Work out the finished part from the listing and answer in its coordinate system (mm). A direction names the side the tool comes from. Round coordinates to 2 decimals unless told otherwise and drop trailing zeros. Write each loop counter-clockwise with the first axis right and the second up, starting at its lowest first coordinate (ties: lowest second). Pieces come first, ordered by that corner, then holes.
from build123d import *

# Parameters (mm, degrees)
BOSS_EXTRUDE1_DEPTH        = 13
CUT_EXTRUDE1_DEPTH         = 71.771362109
CUT_EXTRUDE2_DEPTH         = 62.040693778
F_8_4_8_4_DIAMETER_HOLE1_D = 8.4
CHAMFER2_SIZE              = 9
CHAMFER2_SIZE2             = 8.410167494
CHAMFER3_SIZE              = 8
CHAMFER3_SIZE2             = 8.56106612
SKETCH11_R                 = 4.2
CUT_EXTRUDE5_DEPTH         = 10
CHAMFER4_SIZE              = 0.5
SKETCH12_W                 = 893.834484117
SKETCH12_H                 = 134.722779032
CUT_EXTRUDE6_DEPTH         = 73.047156948


with BuildPart() as part:
    # Sketch1 → Boss-Extrude1 (new body)
    with BuildSketch(Plane(origin=(0, 0, 0), x_dir=(-1, 0, 0), z_dir=(0, 0, -1))):
        with BuildLine():
            Line((-14.999999535, -11.339745693), (-14.999999535, -27.999999731))
            ThreePointArc((-14.999999535, -27.999999731), (4.65e-07, -42.999999731), (15.000000465, -27.999999731))
            Line((15.000000465, -27.999999731), (15.000000465, -13.660253769))
            ThreePointArc((15.000000465, -13.660253769), (16.160254503, -9.33012675), (19.330127484, -6.160253769))
            Line((19.330127484, -6.160253769), (31.748711306, 1.009618943))
            ThreePointArc((31.748711306, 1.009618943), (37.239092363, 6.5), (39.248711306, 14))
            ThreePointArc((39.248711306, 14), (39.245992383, 14.285587643), (39.237836599, 14.571071754))
            Line((39.237836599, 14.571071754), (56.327549631, 24.437822174))
            Line((56.327549631, 24.437822174), (52.827549631, 30.5))
            Line((52.827549631, 30.5), (49.327549631, 36.562177826))
            Line((49.327549631, 36.562177826), (32.237836599, 26.695427407))
            ThreePointArc((32.237836599, 26.695427407), (31.994677998, 26.845232579), (31.748711306, 26.990381057))
            ThreePointArc((31.748711306, 26.990381057), (24.248711306, 29), (16.748711306, 26.990381057))
            Line((16.748711306, 26.990381057), (2.320508541, 18.660254307))
            ThreePointArc((2.320508541, 18.660254307), (-10.358983383, 5.980762382), (-14.999999535, -11.339745693))
        make_face()
    extrude(amount=-BOSS_EXTRUDE1_DEPTH)

    # Sketch2 → Cut-Extrude1 (cut, through all)
    with BuildSketch(Plane(origin=(-7.5, -12.990381057, 0), x_dir=(0.8660254037844388, -0.4999999999999997, 0), z_dir=(-0.4999999999999997, -0.8660254037844388, 0))):
        with BuildLine():
            ThreePointArc((-25.021227161, 9.417565156), (-22, 2.3), (-18.978772839, 9.417565156))
            ThreePointArc((-18.978772839, 9.417565156), (-22, 10.7), (-25.021227161, 9.417565156))
        make_face()
    extrude(amount=-CUT_EXTRUDE1_DEPTH, mode=Mode.SUBTRACT)

    # Sketch3 → Cut-Extrude2 (cut, through all)
    with BuildSketch(Plane.ZY.offset(15.000000465)):
        with BuildLine():
            ThreePointArc((9.417565156, -18.978772839), (2.3, -22), (9.417565156, -25.021227161))
            ThreePointArc((9.417565156, -25.021227161), (10.7, -22), (9.417565156, -18.978772839))
        make_face()
    extrude(amount=-CUT_EXTRUDE2_DEPTH, mode=Mode.SUBTRACT)

    # Ø8.4 (8.4) Diameter Hole1 (through all)
    with Locations(Plane(origin=(0, 0, 0), x_dir=(-1, 0, 0), z_dir=(0, 0, -1))):
        with Locations((29.347432097, 16.831243464), (0.097432097, -33.831242658)):
            Hole(F_8_4_8_4_DIAMETER_HOLE1_D / 2)

    # Chamfer2
    chamfer2_edges = [part.edges().sort_by_distance(p)[0] for p in [
        (-40.782693115, 31.628802617, 0),
    ]]
    chamfer2_side = [part.faces().sort_by_distance(p)[0] for p in [
        (-40.782693115, 31.628802617, 6.5),
    ]]
    chamfer(chamfer2_edges, length=CHAMFER2_SIZE, length2=CHAMFER2_SIZE2, reference=chamfer2_side[0])

    # Chamfer3
    chamfer3_edges = [part.edges().sort_by_distance(p)[0] for p in [
        (-47.782693115, 19.504446964, 13),
    ]]
    chamfer3_side = [part.faces().sort_by_distance(p)[0] for p in [
        (-11.809669845, -1.389258466, 13),
    ]]
    chamfer(chamfer3_edges, length=CHAMFER3_SIZE, length2=CHAMFER3_SIZE2, reference=chamfer3_side[0])

    # Sketch11 → Cut-Extrude5 (cut)
    with BuildSketch(Plane(origin=(-0.376401755, -0.651946963, 0.703467067), x_dir=(-0.9308491020683198, 0.2544179045973002, -0.2622812974630898), z_dir=(0.36532170182252927, 0.6327557486641282, -0.6827592670260799))):
        with Locations(Location((45.831104576, 22.456070648, 0), (0, 0, 89.523216635))):
            Circle(SKETCH11_R)
    extrude(amount=-CUT_EXTRUDE5_DEPTH, mode=Mode.SUBTRACT)

    # Chamfer4
    chamfer4_edges = [part.edges().sort_by_distance(p)[0] for p in [
        (-4.297432097, -33.831242658, 0),
        (-4.297432097, -33.831242658, 13),
        (-33.547432097, 16.831243464, 0),
        (-33.547432097, 16.831243464, 13),
    ]]
    chamfer(chamfer4_edges, length=CHAMFER4_SIZE)

    # Mirror1: part across plane


with BuildPart() as part_1:
    add(part.part)
    add(part.part.mirror(Plane(origin=(0, 0, 0), x_dir=(1, 0, 0), z_dir=(0, 0, -1))))

    # Sketch12 → Cut-Extrude6 (cut, through all)
    with BuildSketch(Plane(origin=(0, 0, 0), x_dir=(-1, 0, 0), z_dir=(0, 0, -1))):
        with Locations((15.524382534, -0.917202718)):
            Rectangle(SKETCH12_W, SKETCH12_H)
    extrude(amount=-CUT_EXTRUDE6_DEPTH, mode=Mode.SUBTRACT)


solid = part_1.part
Q1. Find section B-B (z = -7.75). Count the separate pieces of the cut face and the enclosed holes in it, plus the area to 3 significant figures.
Q2. Find the intervals of material crossed by L1, parallel to Y at x = -3, z = -6.5; L2, parallel to X at y = -27, z = -2.25; L3, parallel to X at y = -31, z = -9.5, in increasing order.
Q3. Find section D-D (x = -35). Determine the outline of the cut face in (y, z), plus the area to 3 significant figures.
Q4. Find section A-A (y = -22). Determine the outline of the cut face in (x, z), plus the area to 3 significant figures.
Q5. Given pin 1 (6 mm diameter, centred on x = -18, y = -34, fed in from +Z); pin 2 (6 mm diameter, centred on y = 26, z = -7.5, fed in from +X); pin 3 (1.5 mm diameter, centred on x = 2, z = -11, fed in from +Y), each flat-ended and moving along its own axis, determine where each tip first touches the part or whether it passes through.
Q6. The mould has two halves that part along X. Classify faces 4 (the face through (15, -17.7, -5)), 5 (the face through (-40.902, 31.698, -10.972)), 6 (the face through (-49.489, 25.044, -8.66)): +X half, -X half, draft (parallel to the pull), parting line (faces both ways), or undercut.
Q7. A tool of negligible diameter and unlimited length cuts with its end or side. For faces 1 (the face through (-15, -17.7, -7.9)), 2 (the face through (-6.429, 21.032, -6.409)), 3 (the face through (-46.83, 30.2, -4.44)), from which of +Z, -Z, +X, -X, +Y, -Y can it reach the whole face along a straight path? Write none if from no direction.
Report:
1. separate pieces: 3
1. enclosed holes: 2
1. area: 1,850 mm2
2. L1: y = -42.7 to -36.87, -30.8 to -26.2, -17.8 to 19.05
2. L2: x = -15 to 15
2. L3: x = -14.7 to -3.2, 3 to 14.7
3. outline: (3.54, -13) - (28.29, -13) - (28.29, -9) - (24.46, -5.45) - (24.46, 0) - (3.54, 0) - close
3. area: 294 mm2
4. outline: (-15, -13) - (15, -13) - (15, -10.7) - (-15, -10.7) - close; (-15, -2.3) - (15, -2.3) - (15, 0) - (-15, 0) - close
4. area: 138 mm2
5. pin 1: passes through
5. pin 2: stops at x = -13.12
5. pin 3: stops at y = 16.29
6. face 4: +X half
6. face 5: undercut
6. face 6: -X half
7. face 1: +Z, -Z, -X, -Y
7. face 2: +Z, -Z, +X, +Y
7. face 3: +Z, +Y
